Geometry: final body of the model. Coordinates: model frame, mm. A direction names the side the tool comes from. Coordinates: 2 decimals unless noted, no trailing zeros. Loops run counter-clockwise (first coordinate to the right, second up) from the corner with the lowest first, then second, coordinate; pieces in that order, holes last. Notation, with made-up numbers: (-15.75, 46.25) - (3.25, 46.25) arc R24 cw to (3.25, 82.25) - close; hole circle Ø11 at (6, 67.25). An arc over 180 degrees is marked (long way). Put each result on its own line as item: value. Start each with the question number.
1) Material intervals for line 1 along Z through (x, y) = (9.15, 1.65); line 2 along X through (y, z) = (0.7, -165.1); line 3 along X through (y, z) = (-2.75, -259.5), sorted ascending. Write a range as from..to.
2) Section B-B on y = -4.25. Output: boundary loops of the cut face in (x, z).
3) Contact query for flat-ended pins moving along their axis: pin 1 Ø3.5 at (x, z) = (9.15, 34.9) entering from -Y; pin 2 Ø5.5 at (x, z) = (5, 8) entering from -Y; pin 3 Ø1.5 at (y, z) = (-13, 85) entering from +X; pin 4 Ø12 at (x, y) = (5, -8.5) entering from -Z. Output: stop coordinate, or through.
4) Reachability of faces 1 (the flat face through (-0.3, -3.4, -305.1)), 2 (the flat face through (0, -9, -4)) from +Z, -Z, +X, -X, +Y, -Y: full face, straight path, thin tool, end or side. Return the list, or none.
5) Section A-A on z = -227. Output: boundary loops of the cut face in (x, y).
Autodesk Inventor part; units mm, degrees
ref_plane "YZ Plane" through (0, 0, 0) normal (1, 0, 0) x (0, 1, 0)
ref_plane "XZ Plane" through (0, 0, 0) normal (0, 1, 0) x (-1, 0, 0)
ref_plane "XY Plane" through (0, 0, 0) normal (0, 0, 1) x (1, 0, 0)
sketch "Esquisse1" plane through (0, 0, 0) normal (0, 0, 1) x (1, 0, 0)
  line L0 (0, 0) -> (18.3, 0)
  line L1 (18.3, 0) -> (18.3, 2.2)
  line L2 (18.3, 2.2) -> (-2.2, 2.2)
  line L3 (-2.2, 2.2) -> (-2.2, -18.3)
  line L4 (-2.2, -18.3) -> (0, -18.3)
  line L5 (0, -18.3) -> (0, 0)
  dimension "Epaisseur_cornière" = 2.2
  dimension "Largueur" = 20.5
extrude "Embase" add sketch "Esquisse1" along normal mid plane 610.2
sketch "Esquisse2" plane through (0, 0, 0) normal (0, 1, 0) x (-1, 0, 0)
  line L0 (2.2, 305.1) -> (-18.3, 284.6)
  line L1 (-18.3, 284.6) -> (-18.3, 305.1)
  line L2 (-18.3, 305.1) -> (2.2, 305.1)
  line L3 (-18.3, 305.1) -> (2.2, 305.1) construction
  line L4 (2.2, -305.1) -> (2.2, 305.1) construction
  line L5 (-18.3, -305.1) -> (-18.3, 305.1) construction
  point P0 (0, 0)
  dimension "d4" = 45
extrude "Découpe à 45" [suppressed]
mirror "Symétrie découpe" [suppressed]
sketch "Esquisse3" plane through (-2.2, 2.2, 305.1) normal (0, 1, 0) x (1, 0, 0)
  line L0 (0, 610.2) -> (20.5, 610.2) construction
  line L1 (20.5, 610.2) -> (20.5, 0) construction
  line L2 (2.2, 0) -> (2.2, 610.2) construction
  point P0 (2.2, 305.1)
  point P1 (11.35, 470.2)
  point P2 (11.35, 456.2)
  dimension "d7" = 14
  dimension "d8" = 140
  dimension "d9" = 9.15
  dimension "d17" = 18.3
hole "Perçage1" at (9.15, 2.2, -165.1) at (9.15, 2.2, -151.1) direction (0, -1, 0) diameter 5.5 end through all
pattern_linear "Réseau rectangulaire1" count 2 spacing 200 along (0, 0, 1) of "Perçage1"
properties part number "1400-06-04 Profilé vertical chaniere" material "Aluminium 6061"
Answer block:
1. line 1: z = -305.1..-167.85, -162.35..-153.85, -148.35..32.15, 37.65..46.15, 51.65..305.1
1. line 2: x = -2.2..6.4, 11.9..18.3
1. line 3: x = -2.2..0
2. outline: (-2.2, -305.1) - (0, -305.1) - (0, 305.1) - (-2.2, 305.1) - close
3. pin 1: passes through
3. pin 2: stops at y = 0
3. pin 3: stops at x = 0
3. pin 4: stops at z = -305.1
4. face 1: -Z, +X, -X, +Y, -Y
4. face 2: +Z, -Z, +X, -Y
5. outline: (-2.2, -18.3) - (0, -18.3) - (0, 0) - (18.3, 0) - (18.3, 2.2) - (-2.2, 2.2) - close
